from build123d import *
from build123d.topology import SkipClean

# Parameters (mm, degrees)
SKETCH_1_W               = 23
SKETCH_1_H               = 23
EXTRUDE_1_DEPTH          = 2
CUT_EXTRUDE_1_DEPTH      = 2
PATTERN_CIRCULAR_1_COUNT = 4
FILLET_1_R               = 3
SKETCH_3_R               = 4
CUT_EXTRUDE_2_DEPTH      = 2
CUT_EXTRUDE_6_DEPTH      = 1
FILLET_2_R               = 0.5
SKETCH_5_R               = 1.005
CUT_EXTRUDE_7_DEPTH      = 2
PATTERN_CIRCULAR_2_COUNT = 2
EXTRUDE_START            = 1
SKETCH_6_R               = 3
SKETCH_6_R_2             = 1.35
EXTRUDE_2_DEPTH          = 1


with BuildPart() as part:
    # Sketch 1 → Extrude 1 (new body)
    with BuildSketch(Plane(origin=(0, 0, 0), x_dir=(1, 0, 0), z_dir=(0, 1, 0))):
        Rectangle(SKETCH_1_W, SKETCH_1_H)
    extrude(amount=EXTRUDE_1_DEPTH)

    # Sketch 2 → Cut-Extrude 1 (cut)
    with BuildSketch(Plane(origin=(0, 2, 0), x_dir=(1, 0, 0), z_dir=(0, 1, 0))):
        with BuildLine():
            ThreePointArc((9.85, -8.5), (9.454594, -7.545406), (8.5, -7.15))
            Line((8.5, -7.15), (8.5, -8.5))
            Line((8.5, -8.5), (7.15, -8.5))
            ThreePointArc((7.15, -8.5), (8.5, -9.85), (9.85, -8.5))
        make_face()
        with BuildLine():
            Line((8.5, -8.5), (8.5, -7.15))
            ThreePointArc((8.5, -7.15), (7.545406, -7.545406), (7.15, -8.5))
            Line((7.15, -8.5), (8.5, -8.5))
        make_face()
        with BuildLine():
            ThreePointArc((9.85, -8.5), (9.454594, -7.545406), (8.5, -7.15))
            Line((8.5, -7.15), (8.5, -8.5))
            Line((8.5, -8.5), (7.15, -8.5))
            ThreePointArc((7.15, -8.5), (8.5, -9.85), (9.85, -8.5))
        make_face()
        with BuildLine():
            Line((8.5, -8.5), (8.5, -7.15))
            ThreePointArc((8.5, -7.15), (7.545406, -7.545406), (7.15, -8.5))
            Line((7.15, -8.5), (8.5, -8.5))
        make_face()
    cut_extrude_1 = extrude(amount=-CUT_EXTRUDE_1_DEPTH, mode=Mode.SUBTRACT)

    # Pattern Circular 1: Cut-Extrude 1 ×4 about axis
    pattern_circular_1_axis = Axis((0, 0, 0), (0, 1, 0))
    for i in range(1, PATTERN_CIRCULAR_1_COUNT):
        add(cut_extrude_1.rotate(pattern_circular_1_axis, i * 360 / PATTERN_CIRCULAR_1_COUNT), mode=Mode.SUBTRACT)

    # Fillet 1
    fillet_1_edges = [part.edges().sort_by_distance(p)[0] for p in [
        (11.5, 1, 11.5),
        (-11.5, 1, 11.5),
        (-11.5, 1, -11.5),
        (11.5, 1, -11.5),
    ]]
    fillet(fillet_1_edges, radius=FILLET_1_R)

    # Sketch 3 → Cut-Extrude 2 (cut)
    with BuildSketch(Plane(origin=(0, 2, 0), x_dir=(1, 0, 0), z_dir=(0, 1, 0))):
        with Locations(Location((0, 0, 0), (0, 0, 270))):
            Circle(SKETCH_3_R)
    extrude(amount=-CUT_EXTRUDE_2_DEPTH, mode=Mode.SUBTRACT)

    # Sketch 4 → Cut-Extrude 6 (cut)
    with SkipClean():  # the faces are left unmerged after this step: merging them gives an invalid solid
        with BuildSketch(Plane(origin=(0, 2, 0), x_dir=(1, 0, 0), z_dir=(0, 1, 0))):
            with BuildLine():
                ThreePointArc((-5.5, -8.5), (-6.37868, -10.62132), (-8.5, -11.5))
                Line((-8.5, -11.5), (8.5, -11.5))
                ThreePointArc((8.5, -11.5), (6.37868, -6.37868), (11.5, -8.5))
                Line((11.5, -8.5), (11.5, 8.5))
                ThreePointArc((11.5, 8.5), (6.37868, 6.37868), (8.5, 11.5))
                Line((8.5, 11.5), (-8.5, 11.5))
                ThreePointArc((-8.5, 11.5), (-6.37868, 10.62132), (-5.5, 8.5))
                ThreePointArc((-5.5, 8.5), (-8.5, 5.5), (-11.5, 8.5))
                Line((-11.5, 8.5), (-11.5, -8.5))
                ThreePointArc((-11.5, -8.5), (-8.5, -5.5), (-5.5, -8.5))
            make_face()
            Polygon((-5, 4), (-5, 0), (-5, -4), (-8.5, -4), (-8.5, 4), align=None, mode=Mode.SUBTRACT)
            with BuildLine():
                ThreePointArc((4, 0), (0, -4), (-4, 0))
                ThreePointArc((-4, 0), (0, 4), (4, 0))
            make_face(mode=Mode.SUBTRACT)
            Polygon((5, -4), (5, 0), (5, 4), (8.5, 4), (8.5, -4), align=None, mode=Mode.SUBTRACT)
        extrude(amount=-CUT_EXTRUDE_6_DEPTH, mode=Mode.SUBTRACT)

    # Fillet 2
    fillet_2_edges = [part.edges().sort_by_distance(p)[0] for p in [
        (-5, 1.5, -4),
        (-8.5, 1.5, -4),
        (-8.5, 1.5, 4),
        (5, 1.5, 4),
        (8.5, 1.5, 4),
        (8.5, 1.5, -4),
        (5, 1.5, -4),
        (-5, 1.5, 4),
    ]]
    fillet(fillet_2_edges, radius=FILLET_2_R)

    # Sketch 5 → Cut-Extrude 7 (cut)
    with SkipClean():  # the faces are left unmerged after this step: merging them gives an invalid solid
        with BuildSketch(Plane(origin=(0, 2, 0), x_dir=(1, 0, 0), z_dir=(0, 1, 0))):
            with Locations(Location((6, 0, 0), (0, 0, 270))):
                Circle(SKETCH_5_R)
        cut_extrude_7 = extrude(amount=-CUT_EXTRUDE_7_DEPTH, mode=Mode.SUBTRACT)

    # Pattern Circular 2: Cut-Extrude 7 ×2 about axis
    with SkipClean():  # the faces are left unmerged after this step: merging them gives an invalid solid
        pattern_circular_2_axis = Axis((0, 0, 0), (0, 1, 0))
        for i in range(1, PATTERN_CIRCULAR_2_COUNT):
            add(cut_extrude_7.rotate(pattern_circular_2_axis, i * 360 / PATTERN_CIRCULAR_2_COUNT), mode=Mode.SUBTRACT)

    # Sketch 6 → Extrude 2 (add)
    # profile 1 of 4: a face of its own
    with BuildSketch(Plane(origin=(0, 2, 0), x_dir=(1, 0, 0), z_dir=(0, 1, 0)).offset(EXTRUDE_START)):
        with Locations(Location((-8.5, -8.5, 0), (0, 0, 270))):
            Circle(SKETCH_6_R)
        with Locations(Location((-8.5, -8.5, 0), (0, 0, 270))):
            Circle(SKETCH_6_R_2, mode=Mode.SUBTRACT)
    # profile 2 of 4: a face of its own
    with BuildSketch(Plane(origin=(0, 2, 0), x_dir=(1, 0, 0), z_dir=(0, 1, 0)).offset(EXTRUDE_START)):
        with Locations(Location((8.5, -8.5, 0), (0, 0, 270))):
            Circle(SKETCH_6_R)
        with Locations(Location((8.5, -8.5, 0), (0, 0, 270))):
            Circle(SKETCH_6_R_2, mode=Mode.SUBTRACT)
    # profile 3 of 4: a face of its own
    with BuildSketch(Plane(origin=(0, 2, 0), x_dir=(1, 0, 0), z_dir=(0, 1, 0)).offset(EXTRUDE_START)):
        with Locations(Location((8.5, 8.5, 0), (0, 0, 90))):
            Circle(SKETCH_6_R)
        with Locations(Location((8.5, 8.5, 0), (0, 0, 270))):
            Circle(SKETCH_6_R_2, mode=Mode.SUBTRACT)
    # profile 4 of 4: a face of its own
    with BuildSketch(Plane(origin=(0, 2, 0), x_dir=(1, 0, 0), z_dir=(0, 1, 0)).offset(EXTRUDE_START)):
        with Locations(Location((-8.5, 8.5, 0), (0, 0, 90))):
            Circle(SKETCH_6_R)
        with Locations(Location((-8.5, 8.5, 0), (0, 0, 270))):
            Circle(SKETCH_6_R_2, mode=Mode.SUBTRACT)
    extrude(amount=-EXTRUDE_2_DEPTH)


solid = part.part
Design review of the part built by this model. Coordinates are the model's own, in mm. A direction names the side the tool comes from. Round coordinates to 2 decimals unless told otherwise and drop trailing zeros. Loops run counter-clockwise (first coordinate to the right, second up) from the corner with the lowest first, then second, coordinate; pieces in that order, holes last. Notation, with made-up numbers: (-8, 78.25) - (35, 78.25) arc R18 cw to (35, 109.25) - close; hole circle Ø7 at (29.25, 70). An arc over 180 degrees is marked (long way). One line per question, with ' | ' between items.
1. For L1, parallel to X at y = 2.4, z = -8.5; L2, parallel to X at y = 0.95, z = 0 (3 decimals), list the stretches that pass through material, from the lowest coordinate up. Write a range as [from, to].
Results are:
L1: x = [-11.5, -9.85], [-7.15, -5.5], [5.5, 7.15], [9.85, 11.5] | L2: x = [-11.5, -7.005], [-4.995, -4], [4, 4.995], [7.005, 11.5]
2. Draft analysis for pull direction Z (two halves, no side actions). For faces 1 (the face through (-0.1, 0.5, 11.5)), 2 (the face through (-0.1, 0.5, -11.5)), 3 (the face through (0, 1, -5)), 4 (the face through (0, 0, 5)), state which applies: released by +Z, released by -Z, zero draft, split by the parting line, or undercut.
Results are:
face 1: released by +Z | face 2: released by -Z | face 3: undercut | face 4: zero draft
3. We need section B-B, the plane y = 0.35. State the section outline as (x, z) points (3 decimals), and give its area (3 significant figures).
Results are:
outline: (-11.5, -8.5) arc R3 ccw to (-8.5, -11.5) - (8.5, -11.5) arc R3 ccw to (11.5, -8.5) - (11.5, 8.5) arc R3 ccw to (8.5, 11.5) - (-8.5, 11.5) arc R3 ccw to (-11.5, 8.5) - close; hole (-8.5, -7.15) arc R1.35 ccw (long way) to (-7.15, -8.5) arc R1.35 ccw to start; hole (-8.5, 7.15) arc R1.35 ccw to (-7.15, 8.5) arc R1.35 ccw (long way) to start; hole circle Ø2.01 at (-6, 0); hole circle Ø8 at (0, 0); hole circle Ø2.01 at (6, 0); hole (7.15, -8.5) arc R1.35 ccw (long way) to (8.5, -7.15) arc R1.35 ccw to start; hole (7.15, 8.5) arc R1.35 ccw to (8.5, 7.15) arc R1.35 ccw (long way) to start | area: 442 mm²
4. For faces 5 (the face through (-8, 3, -10)), 6 (the face through (-8.5, 1.5, 0)), 7 (the face through (-5, 1.5, -1.8)), 8 (the face through (-5.39, 1.01, 0.8)), 9 (the face through (-6.8, 1.5, -4)), list the 3-axis set-ups (+Z, -Z, +X, -X, +Y, -Y) from which the entire face can be reached by the end or side of a thin tool; tool diameter is ignored.
Results are:
face 5: +Z, -Z, +X, -X, +Y | face 6: -X, +Y | face 7: +Z, -Z, +Y | face 8: +Y, -Y | face 9: +X, -X, +Y
5. We need section D-D, the plane z = 9.5. State the section outline as (x, y) points.
Results are:
outline: (-11.33, 0) - (-9.41, 0) - (-9.41, 3) - (-11.33, 3) - close; (-7.59, 0) - (7.59, 0) - (7.59, 3) - (5.67, 3) - (5.67, 1) - (-5.67, 1) - (-5.67, 3) - (-7.59, 3) - close; (9.41, 0) - (11.33, 0) - (11.33, 3) - (9.41, 3) - close
6. We need section A-A, the plane x = 0. State the section outline as (y, z) points, and give its area (3 significant figures).
Results are:
outline: (0, -11.5) - (1, -11.5) - (1, -4) - (0, -4) - close; (0, 4) - (1, 4) - (1, 11.5) - (0, 11.5) - close | area: 15.0 mm²
7. Clearance check with flat-ended pins moving along their axes: P1, Ø0.8, axis at y = 1.5, z = -1, coming from the -X side; P2, Ø0.5, axis at x = -6.5, y = 1.5, coming from the -Z side; P3, Ø4, axis at x = -5.5, z = -3, coming from the +Y side; P4, Ø1.6, axis at x = 6, z = 0, coming from the +Y side. State where each tip first meets the part, or that it passes through.
Results are:
P1: stops at x = -8.5 | P2: stops at z = -10.94 | P3: stops at y = 2 | P4: passes through
8. We need section C-C, the plane x = 9. State the section outline as (y, z) points, and give its area (3 significant figures).
Results are:
outline: (0, -11.46) - (3, -11.46) - (3, -9.75) - (0, -9.75) - close; (0, -7.25) - (3, -7.25) - (3, -5.54) - (1, -5.54) - (1, 5.54) - (3, 5.54) - (3, 7.25) - (0, 7.25) - close; (0, 9.75) - (3, 9.75) - (3, 11.46) - (0, 11.46) - close | area: 31.5 mm²
